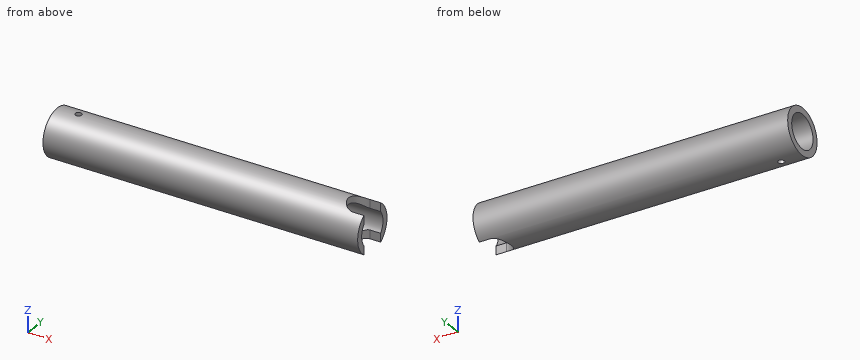
Autodesk Inventor part; units mm, degrees
ref_plane "YZ Plane" through (0, 0, 0) normal (1, 0, 0) x (0, 1, 0)
ref_plane "XZ Plane" through (0, 0, 0) normal (0, 1, 0) x (-1, 0, 0)
ref_plane "XY Plane" through (0, 0, 0) normal (0, 0, 1) x (1, 0, 0)
sketch "スケッチ1" plane through (0, 0, 0) normal (1, 0, 0) x (0, 1, 0)
  circle A0 centre (0, 0) radius 11
  circle A1 centre (0, 0) radius 8
  dimension "d0" = 22
  dimension "d1" = 16
extrude "押し出し1" add sketch "スケッチ1" against normal blind 150
sketch "スケッチ2" plane through (0, 0, 0) normal (0, 0, 1) x (1, 0, 0)
  line L0 (0, 0) -> (0, 6.25)
  line L1 (0, 8) -> (0, -8)
  line L2 (0, 0) -> (0, -6.25)
  line L3 (0, -6.25) -> (-5, -6.25)
  line L4 (-5, -6.25) -> (-5, 6.25)
  line L5 (-5, 6.25) -> (0, 6.25)
  dimension "d4" = 6.25
  dimension "d5" = 6.25
  dimension "d6" = 5
extrude "押し出し2" cut sketch "スケッチ2" along normal mid plane 150
sketch "スケッチ3" plane through (0, 0, 0) normal (0, 0, 1) x (1, 0, 0)
  line L0 (-5, -6.25) -> (-5, 6.25)
  line L1 (-5, 6.25) -> (0, 6.25)
  circle A0 centre (-5, 0) radius 6.25
  point P0 (0, 0)
extrude "押し出し3" cut sketch "スケッチ3" along normal mid plane 150 contours A0 L0 picked at (-7.0681, 0.2511)
sketch "スケッチ4" plane through (0, 0, 0) normal (0, 0, 1) x (1, 0, 0)
  circle A0 centre (-140, 0) radius 1.5
  point P0 (0, 0)
  dimension "d11" = 3
extrude "押し出し4" cut sketch "スケッチ4" along normal mid plane 150
thread "ねじ1"
thread "ねじ2"
properties part number "VP16_200" material "PVC 配管"
Check sheet for the modelled part. Datum: model origin and axes. Units: mm. Round coordinates to 2 decimals unless told otherwise and drop trailing zeros. Order: outer loops, then holes, each group sorted by start corner. A loop starts at its lowest first (then second) coordinate and runs counter-clockwise, first axis right, second up. Notation, with made-up numbers: (27, 66) - (67, 66) arc R20 cw to (67, 96) - close; hole circle Ø9 at (-3.5, -1). An arc over 180 degrees is marked (long way). Write item = value, one per line.
Q1. Thickness scan on line 1 along Y through (x, z) = (-124.5, 0); line 2 along X through (y, z) = (0, 8.95). Record the ranges inside material, lowest first.
Computed:
line_1 = -11 to -8, 8 to 11
line_2 = -150 to -141.5, -138.5 to -11.25
Q2. Section check C-C (x = -140). Record the boundary of the cut face in (y, z).
Computed:
outline = (-1.5, -10.9) - (-1.5, -7.86) arc R8 cw to (-1.5, 7.86) - (-1.5, 10.9) arc R11 ccw to start; (1.5, -10.9) arc R11 ccw to (1.5, 10.9) - (1.5, 7.86) arc R8 cw to (1.5, -7.86) - close
Q3. Go/stop test with flat-tipped pins: pin 1 (1.5 mm diameter, centred on x = -16, y = 5.5, fed in from -Z); pin 2 (6 mm diameter, centred on x = -94, y = -5.5, fed in from +Z); pin 3 (4 mm diameter, centred on x = -33.5, y = -5, fed in from +Z). Record where each tip stops, or that it passes through.
Computed:
pin_1 = -9.92
pin_2 = 10.71
pin_3 = 10.58
Q4. Section check D-D (x = -52.5). Record the boundary of the cut face in (y, z).
Computed:
outline = circle Ø22 at (0, 0); hole circle Ø16 at (0, 0)
Q5. Section check B-B (z = -3.75). Record the boundary of the cut face in (x, y).
Computed:
outline = (-150, -10.34) - (0, -10.34) - (0, -7.07) - (-150, -7.07) - close; (-150, 7.07) - (0, 7.07) - (0, 10.34) - (-150, 10.34) - close
Q6. Section check A-A (y = 0). Record the boundary of the cut face in (x, z), and give its area (4 significant figures).
Computed:
outline = (-150, -11) - (-141.5, -11) - (-141.5, -8) - (-150, -8) - close; (-150, 8) - (-141.5, 8) - (-141.5, 11) - (-150, 11) - close; (-138.5, -11) - (-11.25, -11) - (-11.25, -8) - (-138.5, -8) - close; (-138.5, 8) - (-11.25, 8) - (-11.25, 11) - (-138.5, 11) - close
area = 814.5 mm^2
